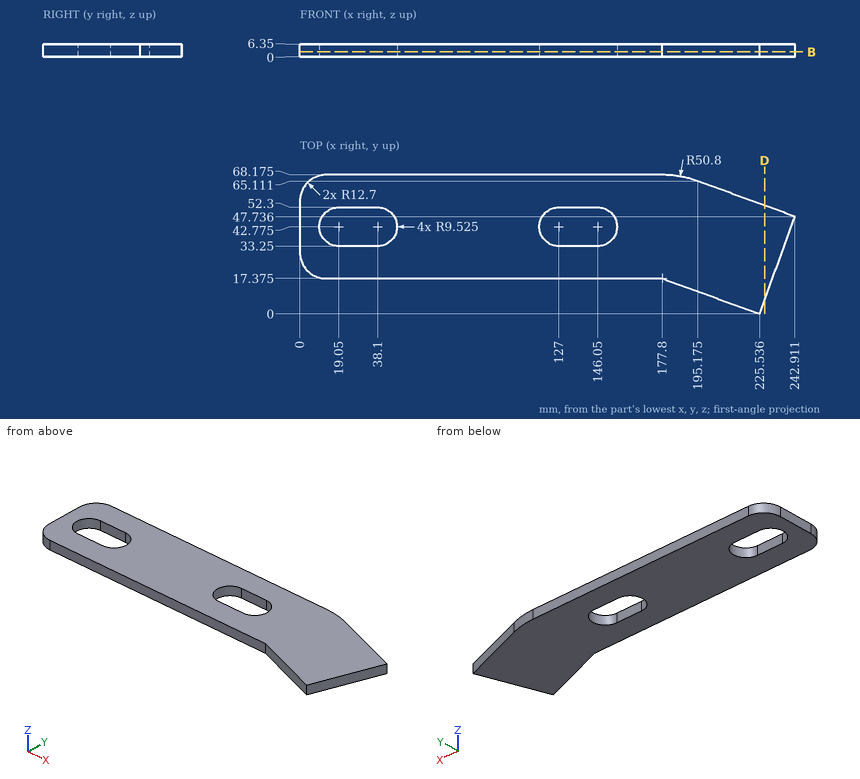
Geometry check sheet. Reference: drawing and pictorial views, mm from the part's lowest x, y, z. Coordinates: 2 decimals unless noted, no trailing zeros. Write each loop counter-clockwise with the first axis right and the second up, starting at its lowest first coordinate (ties: lowest second). Pieces come first, ordered by that corner, then holes. Notation, with made-up numbers: M 5,-4.75 L 64,-4.75 A16 cw 64,3.25 Z; hole C 59.25,-7 d4. An arc over 180 degrees is marked long. One line per question, with ' | ' between items.
1) Sectioned sample at D-D on x = 228. Record the cut outline in (y, z).
Solutions:
outline: M 6.77,0 L 53.16,0 L 53.16,6.35 L 6.77,6.35 Z
2) Material ranges on L1, parallel to X at y = 47.5, z = 1.25 (1 decimal); L2, parallel to X at y = 47, z = 5.5 (1 decimal); L3, parallel to Y at x = 171.5, z = 3.5 (1 decimal), recorded low to high.
Solutions:
L1: 0 to 10.8, 46.4 to 118.7, 154.3 to 242.8 | L2: 0 to 10.5, 46.6 to 118.5, 154.6 to 242.6 | L3: 17.4 to 68.2
3) Depth check by flat-ended pin: pin 1 Ø1.5 at (x, z) = (62, 1) entering from -Y (1 decimal). Enter the tip coordinate at first touch or a pass-through.
Solutions:
pin 1: y = 17.4
4) Sectioned sample at B-B on z = 2.5. State how many separate pieces and enclosed holes the cut face has, then the cut area to 3 significant figures.
Solutions:
separate pieces: 1 | enclosed holes: 2 | area: 10,700 mm^2
